from build123d import *

# Parameters (mm, degrees)
SKETCH1_W                   = 24
SKETCH1_H                   = 6
BOSS_EXTRUDE1_DEPTH         = 27
CUT_EXTRUDE1_DEPTH          = 27
BOSS_EXTRUDE2_DEPTH         = 1
SKETCH4_W                   = 3
SKETCH4_H                   = 1
CUT_EXTRUDE2_DEPTH          = 8
FILLET1_R                   = 1
SKETCH5_W                   = 14
SKETCH5_H                   = 40
BOSS_EXTRUDE3_DEPTH         = 1
BOSS_EXTRUDE4_DEPTH         = 1
FILLET2_R                   = 14
SKETCH6_W                   = 1.5
SKETCH6_H                   = 3.5
CUT_EXTRUDE3_DEPTH          = 3
TAP_DRILL_FOR_M3X0_5_TAP1_D = 2.5
FILLET3_R                   = 0.5


with BuildPart() as part:
    # Sketch1 → Boss-Extrude1 (new body)
    with BuildSketch(Plane(origin=(0, 0, 0), x_dir=(1, 0, 0), z_dir=(0, 1, 0))):
        with Locations((12, 3)):
            Rectangle(SKETCH1_W, SKETCH1_H)
    extrude(amount=BOSS_EXTRUDE1_DEPTH)

    # Sketch2 → Cut-Extrude1 (cut)
    with BuildSketch(Plane(origin=(0, 27, 0), x_dir=(1, 0, 0), z_dir=(0, 1, 0))):
        Polygon((1, 1), (23, 1), (23, 5), (20, 5), (20, 7.622720443), (4, 7.622720443), (4, 5), (1, 5), align=None)
    extrude(amount=-CUT_EXTRUDE1_DEPTH, mode=Mode.SUBTRACT)

    # Sketch3 → Boss-Extrude2 (add)
    with BuildSketch(Plane(origin=(0, 27, 0), x_dir=(1, 0, 0), z_dir=(0, 1, 0))):
        Polygon((24, 0), (24, 5), (24, 6), (20, 6), (20, 5), (4, 5), (4, 6), (0, 6), (0, 5), (0, 0), align=None)
    extrude(amount=BOSS_EXTRUDE2_DEPTH)

    # Sketch4 → Cut-Extrude2 (cut)
    with BuildSketch(Plane.XZ):
        with Locations((2.5, -5.5)):
            Rectangle(SKETCH4_W, SKETCH4_H)
        with Locations((21.5, -5.5)):
            Rectangle(SKETCH4_W, SKETCH4_H)
    extrude(amount=-CUT_EXTRUDE2_DEPTH, mode=Mode.SUBTRACT)

    # Fillet1
    fillet1_edges = [part.edges().sort_by_distance(p)[0] for p in [
        (1, 8, -5.5),
        (23, 8, -5.5),
    ]]
    fillet(fillet1_edges, radius=FILLET1_R)

    # Sketch5 → Boss-Extrude3 (add)
    with BuildSketch(Plane.XY):
        with Locations((12, -20)):
            Rectangle(SKETCH5_W, SKETCH5_H)
    extrude(amount=-BOSS_EXTRUDE3_DEPTH)

    # Sketch7 → Boss-Extrude4 (add)
    with BuildSketch(Plane.XY):
        Polygon((0, 28), (0, 0), (5, 0), (5, -40), (19, -40), (19, 0), (24, 0), (24, 28), align=None)
    extrude(amount=BOSS_EXTRUDE4_DEPTH)

    # Fillet2
    # the kernel refuses this fillet: 14 mm, written as the material it adds along each edge
    with BuildSketch(Plane(origin=(19, 0, -27.809513237), x_dir=(0, -1, 0), z_dir=(0, 0, 1))) as fillet2_piece_1_section:
        with BuildLine():
            CenterArc((10.723805295, 14), FILLET2_R, 220.005200885, 49.994799115)
            Line((0, 5), (-0.214476106, 4.82))
            ThreePointArc((-0.214476106, 4.82), (-0.28, 2.5), (-0.28, 0))
            Line((-0.28, 0), (0, -0.28))
            Line((0, -0.28), (10.723805295, -0.28))
            Line((10.723805295, -0.28), (10.723805295, 0))
        make_face()
    fillet2_piece_1 = extrude(amount=28.809513237, mode=Mode.PRIVATE)
    fillet2_piece_1 = split(fillet2_piece_1, bisect_by=Plane(origin=(23.365169803, -0.171945875, -1), z_dir=(0, 0, -1)), keep=Keep.TOP, mode=Mode.PRIVATE)
    fillet2_piece_1 = split(fillet2_piece_1, bisect_by=Plane(origin=(23.365169803, -0.171945875, -6), z_dir=(0, 0, 1)), keep=Keep.TOP, mode=Mode.PRIVATE)
    fillet2_piece_1 = split(fillet2_piece_1, bisect_by=Plane(origin=(23, -0.171945875, -3.5), z_dir=(1, 0, 0)), keep=Keep.TOP, mode=Mode.PRIVATE)
    add(fillet2_piece_1)
    with BuildSketch(Plane(origin=(19, 0, -1), x_dir=(0, -1, 0), z_dir=(0, 0, 1))) as fillet2_piece_2_section:
        with BuildLine():
            CenterArc((10.723805295, 14), FILLET2_R, 220.005200885, 49.994799115)
            Line((0, 5), (-0.214476106, 4.82))
            ThreePointArc((-0.214476106, 4.82), (-0.28, 2.5), (-0.28, 0))
            Line((-0.28, 0), (0, -0.28))
            Line((0, -0.28), (10.723805295, -0.28))
            Line((10.723805295, -0.28), (10.723805295, 0))
        make_face()
    fillet2_piece_2 = extrude(amount=2, mode=Mode.PRIVATE)
    fillet2_piece_2 = split(fillet2_piece_2, bisect_by=Plane(origin=(23, -2.887653154, 0), z_dir=(-1, 0, 0)), keep=Keep.TOP, mode=Mode.PRIVATE)
    add(fillet2_piece_2)
    with BuildSketch(Plane(origin=(19, 0, -1), x_dir=(0, -1, 0), z_dir=(0, 0, 1))) as fillet2_piece_3_section:
        with BuildLine():
            CenterArc((10.723805295, 14), FILLET2_R, 220.005200885, 49.994799115)
            Line((0, 5), (-0.214476106, 4.82))
            ThreePointArc((-0.214476106, 4.82), (-0.28, 2.5), (-0.28, 0))
            Line((-0.28, 0), (0, -0.28))
            Line((0, -0.28), (10.723805295, -0.28))
            Line((10.723805295, -0.28), (10.723805295, 0))
        make_face()
    fillet2_piece_3 = extrude(amount=2, mode=Mode.PRIVATE)
    fillet2_piece_3 = split(fillet2_piece_3, bisect_by=Plane(origin=(23, -0.171945875, 0), z_dir=(1, 0, 0)), keep=Keep.TOP, mode=Mode.PRIVATE)
    add(fillet2_piece_3)
    with BuildSketch(Plane(origin=(5, 0, -27.809513237), x_dir=(-1, 0, 0), z_dir=(0, 0, 1))) as fillet2_piece_4_section:
        with BuildLine():
            CenterArc((14, 10.723805295), FILLET2_R, 180, 49.994799115)
            Line((0, 10.723805295), (-0.28, 10.723805295))
            Line((-0.28, 10.723805295), (-0.28, 0))
            Line((-0.28, 0), (0, -0.28))
            ThreePointArc((0, -0.28), (2.5, -0.28), (4.82, -0.214476106))
            Line((4.82, -0.214476106), (5, 0))
        make_face()
    fillet2_piece_4 = extrude(amount=28.809513237, mode=Mode.PRIVATE)
    fillet2_piece_4 = split(fillet2_piece_4, bisect_by=Plane(origin=(1, -0.171945875, -3.5), z_dir=(-1, 0, 0)), keep=Keep.TOP, mode=Mode.PRIVATE)
    fillet2_piece_4 = split(fillet2_piece_4, bisect_by=Plane(origin=(0.634830197, -0.171945875, -6), z_dir=(0, 0, 1)), keep=Keep.TOP, mode=Mode.PRIVATE)
    fillet2_piece_4 = split(fillet2_piece_4, bisect_by=Plane(origin=(0.634830197, -0.171945875, -1), z_dir=(0, 0, -1)), keep=Keep.TOP, mode=Mode.PRIVATE)
    add(fillet2_piece_4)
    with BuildSketch(Plane(origin=(5, 0, -1), x_dir=(-1, 0, 0), z_dir=(0, 0, 1))) as fillet2_piece_5_section:
        with BuildLine():
            CenterArc((14, 10.723805295), FILLET2_R, 180, 49.994799115)
            Line((0, 10.723805295), (-0.28, 10.723805295))
            Line((-0.28, 10.723805295), (-0.28, 0))
            Line((-0.28, 0), (0, -0.28))
            ThreePointArc((0, -0.28), (2.5, -0.28), (4.82, -0.214476106))
            Line((4.82, -0.214476106), (5, 0))
        make_face()
    fillet2_piece_5 = extrude(amount=2, mode=Mode.PRIVATE)
    fillet2_piece_5 = split(fillet2_piece_5, bisect_by=Plane(origin=(1, -0.171945875, 0), z_dir=(-1, 0, 0)), keep=Keep.TOP, mode=Mode.PRIVATE)
    add(fillet2_piece_5)
    with BuildSketch(Plane(origin=(5, 0, -1), x_dir=(-1, 0, 0), z_dir=(0, 0, 1))) as fillet2_piece_6_section:
        with BuildLine():
            CenterArc((14, 10.723805295), FILLET2_R, 180, 49.994799115)
            Line((0, 10.723805295), (-0.28, 10.723805295))
            Line((-0.28, 10.723805295), (-0.28, 0))
            Line((-0.28, 0), (0, -0.28))
            ThreePointArc((0, -0.28), (2.5, -0.28), (4.82, -0.214476106))
            Line((4.82, -0.214476106), (5, 0))
        make_face()
    fillet2_piece_6 = extrude(amount=2, mode=Mode.PRIVATE)
    fillet2_piece_6 = split(fillet2_piece_6, bisect_by=Plane(origin=(1, -2.887653154, 0), z_dir=(1, 0, 0)), keep=Keep.TOP, mode=Mode.PRIVATE)
    add(fillet2_piece_6)

    # Sketch6 → Cut-Extrude3 (cut)
    with BuildSketch(Plane(origin=(0, 0, -1), x_dir=(-1, 0, 0), z_dir=(0, 0, -1))):
        with Locations((-6.986389138, -35.987474117)):
            Rectangle(SKETCH6_W, SKETCH6_H)
        with Locations((-16.986389138, -35.987474117)):
            Rectangle(SKETCH6_W, SKETCH6_H)
        with Locations((-6.986389138, -25.987474117)):
            Rectangle(SKETCH6_W, SKETCH6_H)
        with Locations((-16.986389138, -25.987474117)):
            Rectangle(SKETCH6_W, SKETCH6_H)
        with Locations((-16.986389138, -15.987474117)):
            Rectangle(SKETCH6_W, SKETCH6_H)
        with Locations((-6.986389138, -15.987474117)):
            Rectangle(SKETCH6_W, SKETCH6_H)
    extrude(amount=-CUT_EXTRUDE3_DEPTH, mode=Mode.SUBTRACT)

    # Tap Drill for M3x0.5 Tap1 (through all)
    with Locations(Plane.XY.offset(1)):
        with Locations((11.986389138, -30.987474117)):
            Hole(TAP_DRILL_FOR_M3X0_5_TAP1_D / 2)

    # Fillet3
    fillet3_edges = [part.edges().sort_by_distance(p)[0] for p in [
        (23, -0.925846324, -3.5),
        (1, -0.925846324, -3.5),
        (4, 8, -5.5),
        (20, 8, -5.5),
    ]]
    fillet(fillet3_edges, radius=FILLET3_R)


solid = part.part
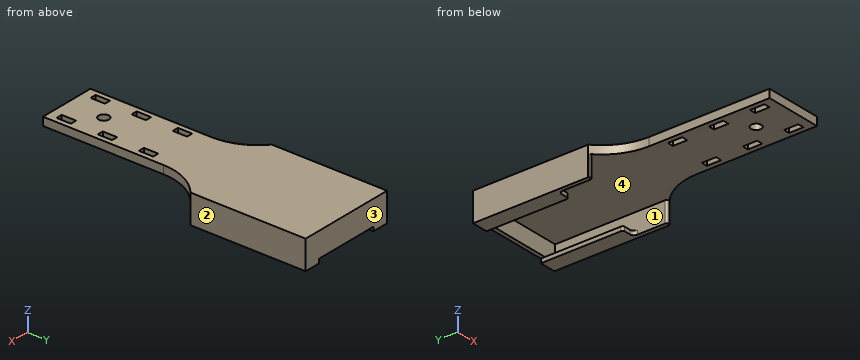
Verification items for the finished model (mm, model axes). Face numbers are marked on the shaded views. Coordinates: 2 decimals unless noted, no trailing zeros. Write each loop counter-clockwise with the first axis right and the second up, starting at its lowest first coordinate (ties: lowest second). Pieces come first, ordered by that corner, then holes. Notation, with made-up numbers: (-1.75, 27.25) - (11.25, 27.25) arc R16 ccw to (11.25, 46.25) - close; hole circle Ø3 at (-23, -20). An arc over 180 degrees is marked (long way). Answer as a JSON object with one key per item and string values.
(1) Cross-section at A-A on x = 7. Record the cut outline in (y, z).
Report:
{"outline": "(-40, -1) - (-37.74, -1) - (-37.74, 1) - (-40, 1) - close; (-34.24, -1) - (-27.74, -1) - (-27.74, 1) - (-34.24, 1) - close; (-24.24, -1) - (-17.74, -1) - (-17.74, 1) - (-24.24, 1) - close; (-14.24, -1) - (27, -1) - (27, -5) - (28, -5) - (28, 1) - (-14.24, 1) - close"}
(2) Cross-section at B-B on y = 17. Record the cut outline in (x, z), plus the area to 3 significant figures.
Report:
{"outline": "(0, -6) - (4, -6) - (4, -5) - (1, -5) - (1, -1) - (23, -1) - (23, -5) - (20, -5) - (20, -6) - (24, -6) - (24, 1) - (0, 1) - close", "area": "64.0 mm^2"}
(3) Cross-section at C-C on z = -3.5. Record the cut outline in (x, y).
Report:
{"outline": "(0, 0) arc R14 cw to (0.17, -0.15) arc R0.5 ccw to (1, 0.23) - (1, 27) - (23, 27) - (23, 0.23) arc R0.5 ccw to (23.83, -0.15) arc R14 cw to (24, 0) - (24, 28) - (0, 28) - close"}
(4) Thickness scan on line 1 along X through (y, z) = (-25, 0.5); line 2 along Y through (x, z) = (17.5, 0); line 3 along X through (y, z) = (12, -3.5). Record the ranges inside material, lowest first.
Report:
{"line 1": "5 to 6.24, 7.74 to 16.24, 17.74 to 19", "line 2": "-40 to -37.74, -34.24 to -27.74, -24.24 to -17.74, -14.24 to 28", "line 3": "0 to 1, 23 to 24"}
(5) Gauge pin test, flat ends, axial feed: pin 1 Ø3 at (x, y) = (11.99, -30.99) entering from -Z; pin 2 Ø2 at (y, z) = (-36, 0) entering from -X; pin 3 Ø1.2 at (x, z) = (8, -3.5) entering from -Y. Record the tip position at first contact, or that the pin passes through.
Report:
{"pin 1": "z = -1", "pin 2": "x = 5", "pin 3": "y = 27"}
(6) Mould release check, pull along X, two halves, no side actions. Record for the marked faces 1, 2, 3 and 4: pulls with the +X half, pulls with the -X half, needs draft (parallel to the pull), parting line crosses it, or undercut.
Report:
{"face 1": "undercut", "face 2": "pulls with the +X half", "face 3": "needs draft", "face 4": "undercut"}
(7) Cross-section at D-D on z = 0.25. Give the number of separate pieces and of enclosed holes in the cut face, plus the area to 3 significant figures.
Report:
{"separate pieces": "1", "enclosed holes": "7", "area": "1,230 mm^2"}
